Model file for the job. Use its own axes, mm. Face numbers are marked on the shaded views. A direction names the side the tool comes from. Coordinates: 2 decimals unless noted, no trailing zeros. Order: outer loops, then holes, each group sorted by start corner. A loop starts at its lowest first (then second) coordinate and runs counter-clockwise, first axis right, second up. Notation, with made-up numbers: M -34.5,31 L 3.5,31 A24 ccw 3.5,54 Z; hole C 33.25,48.25 d4. An arc over 180 degrees is marked long. Return JSON: item names as keys, results as strings.
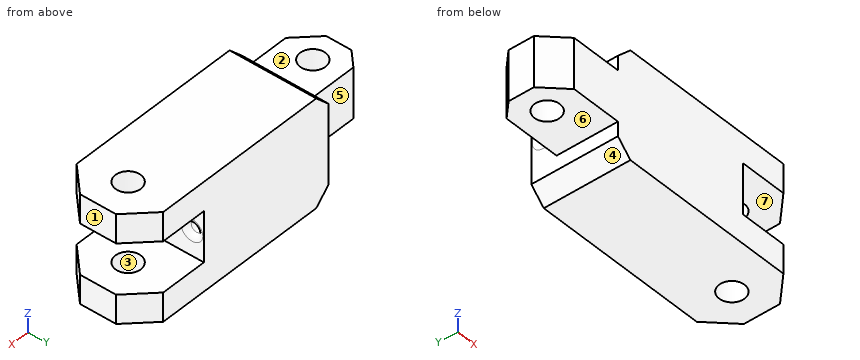
```python
from build123d import *

# Parameters (mm, degrees)
SKETCH_2_W            = 15
SKETCH_2_H            = 12
EXTRUDE_1_DEPTH       = 40
SKETCH_3_W            = 13.345049732
SKETCH_3_H            = 6.461251269
CUT_EXTRUDE_1_DEPTH   = 43.429353047
SKETCH_4_R            = 1.75
CUT_EXTRUDE_2_DEPTH   = 42.91658383
SKETCH_5_W            = 15.367688112
SKETCH_5_H            = 7
CUT_EXTRUDE_2_2_DEPTH = 43.429353047
CHAMFER_4_SIZE        = 3.5
SKETCH_7_R            = 0.75
CUT_EXTRUDE_3_DEPTH   = 32.5
CHAMFER_5_SIZE        = 3
SKETCH_8_W            = 20.918678204
SKETCH_8_H            = 3.864211738
CUT_EXTRUDE_4_DEPTH   = 10
CHAMFER_6_SIZE        = 2
SKETCH_9_R            = 1.75
CUT_EXTRUDE_5_DEPTH   = 44.13930922
FILLET_6_R            = 0.75
CHAMFER_7_SIZE        = 2


with BuildPart() as part:
    # Эскиз2 → Вытянуть1 (new body)
    with BuildSketch(Plane(origin=(0, 0, 0), x_dir=(0, 0, -1), z_dir=(1, 0, 0))):
        Rectangle(SKETCH_2_W, SKETCH_2_H)
    extrude(amount=EXTRUDE_1_DEPTH)

    # Эскиз3 → Вырез-Вытянуть1 (cut, through all)
    with BuildSketch(Plane(origin=(0, 6, 0), x_dir=(1, 0, 0), z_dir=(0, 1, 0))):
        with Locations((3.327475134, -6.730625634)):
            Rectangle(SKETCH_3_W, SKETCH_3_H)
        with Locations((3.327475134, 6.730625634)):
            Rectangle(SKETCH_3_W, SKETCH_3_H)
    extrude(amount=-CUT_EXTRUDE_1_DEPTH, mode=Mode.SUBTRACT)

    # Эскиз4 → Cut-Extrude 2 (cut, through all)
    with BuildSketch(Plane.XY.offset(3.5)):
        with Locations((3.849904433, -1.520907782)):
            Circle(SKETCH_4_R)
    extrude(amount=-CUT_EXTRUDE_2_DEPTH, mode=Mode.SUBTRACT)

    # Эскиз5 → Cut-Extrude 2 2 (cut, through all)
    with BuildSketch(Plane(origin=(0, 6, 0), x_dir=(1, 0, 0), z_dir=(0, 1, 0))):
        with Locations((37.683844056, 0)):
            Rectangle(SKETCH_5_W, SKETCH_5_H)
    extrude(amount=-CUT_EXTRUDE_2_2_DEPTH, mode=Mode.SUBTRACT)

    # Фаска4
    chamfer_4_edges = [part.edges().sort_by_distance(p)[0] for p in [
        (40, -6, 5.5),
        (40, 6, 5.5),
        (40, -6, -5.5),
        (40, 6, -5.5),
    ]]
    chamfer(chamfer_4_edges, length=CHAMFER_4_SIZE)

    # Эскиз7 → Вытянуть3 (cut, through all)
    with BuildSketch(Plane(origin=(30, 0, 0), x_dir=(0, 0, -1), z_dir=(1, 0, 0))):
        with Locations((0, 4.357693323)):
            Circle(SKETCH_7_R)
    extrude(amount=-CUT_EXTRUDE_3_DEPTH, mode=Mode.SUBTRACT)

    # Фаска5
    chamfer_5_edges = [part.edges().sort_by_distance(p)[0] for p in [
        (0, -6, 0),
    ]]
    chamfer(chamfer_5_edges, length=CHAMFER_5_SIZE)

    # Эскиз8 → Вытянуть4 (cut)
    with BuildSketch(Plane.ZY):
        with Locations((-0.939401822, 4.432105869)):
            Rectangle(SKETCH_8_W, SKETCH_8_H)
    extrude(amount=-CUT_EXTRUDE_4_DEPTH, mode=Mode.SUBTRACT)

    # Фаска6
    chamfer_6_edges = [part.edges().sort_by_distance(p)[0] for p in [
        (0, 2.5, 0),
    ]]
    chamfer(chamfer_6_edges, length=CHAMFER_6_SIZE)

    # Эскиз9 → Вытянуть5 (cut, through all)
    with BuildSketch(Plane.XY.offset(7.5)):
        with Locations((35.185724632, 0)):
            Circle(SKETCH_9_R)
    extrude(amount=-CUT_EXTRUDE_5_DEPTH, mode=Mode.SUBTRACT)

    # Скругление6
    fillet_6_edges = [part.edges().sort_by_distance(p)[0] for p in [
        (30, 4.357693323, 0.75),
        (10, 4.357693323, 0.75),
    ]]
    fillet(fillet_6_edges, radius=FILLET_6_R)

    # Фаска7
    chamfer_7_edges = [part.edges().sort_by_distance(p)[0] for p in [
        (10, 0, -7.5),
        (10, 0, 7.5),
    ]]
    chamfer(chamfer_7_edges, length=CHAMFER_7_SIZE)


solid = part.part
```
Item 1: Saw through at D-D (z = 6.75). Write the cut outline in (x, y), and give its area (3 significant figures).
Check result:
{"outline": "M 11.25,-6 L 36.5,-6 L 40,-2.5 L 40,2.5 L 36.5,6 L 11.25,6 Z; hole C 35.19,0 d3.5", "area": "323 mm2"}
Item 2: 3-axis set-ups, long thin cutter, end or side, ignore diameter. For the marked faces 5, 6 and 7: which of +Z, -Z, +X, -X, +Y, -Y reach the whole face in a straight line?
Check result:
{"face 5": "+Z, -Z, -X, +Y", "face 6": "-Z, -X, +Y, -Y", "face 7": "+X, +Y, -Y"}
Item 3: Saw through at B-B (z = -5). Write the cut outline in (x, y).
Check result:
{"outline": "M 10,-6 L 36.5,-6 L 40,-2.5 L 40,2.5 L 36.5,6 L 10,6 Z; hole C 35.19,0 d3.5"}
Item 4: Wall check: line 1 (Z direction, x = 31, y = -1.75); line 2 (Y direction, x = 19.5, z = 0); line 3 (X direction, y = 1.25, z = -0.5). Give the ranges that are in metal, low to high.
Check result:
{"line 1": "z = -7.5 to -3.5, 3.5 to 7.5", "line 2": "y = -6 to 3.61, 5.11 to 6", "line 3": "x = 0.75 to 30"}
Item 5: Saw through at C-C (z = 0). Write the cut outline in (x, y).
Check result:
{"outline": "M 0,-3 L 3,-6 L 30,-6 L 30,2.86 A0.75 ccw 29.25,3.61 L 10.75,3.61 A0.75 ccw 10,2.86 L 10,2.5 L 2,2.5 L 0,0.5 Z; M 10,5.86 A0.75 ccw 10.75,5.11 L 29.25,5.11 A0.75 ccw 30,5.86 L 30,6 L 10,6 Z; hole C 3.85,-1.52 d3.5"}
Item 6: Drop flat-ended pins along their axis: pin 1 Ø4 at (x, y) = (3.85, -1.52) entering from -Z; pin 2 Ø2 at (x, z) = (6.5, 1.5) entering from +Y; pin 3 Ø2 at (y, z) = (2.5, -1) entering from +X. Give the stop position or say it passes through.
Check result:
{"pin 1": "stops at z = -3.5", "pin 2": "stops at y = 2.5", "pin 3": "stops at x = 30"}
Item 7: Pull direction X, two halves, no side cores. Call the marked faces 1, 2, 3 and 4: +X half, -X half, draft (parallel to the pull), parting line (faces both ways), or undercut.
Check result:
{"face 1": "+X half", "face 2": "draft", "face 3": "undercut", "face 4": "-X half"}
Item 8: Saw through at A-A (x = 37.5). Write the cut outline in (y, z), and give its area (3 significant figures).
Check result:
{"outline": "M -5,-7.5 L 5,-7.5 L 5,-3.5 L -5,-3.5 Z; M -5,3.5 L 5,3.5 L 5,7.5 L -5,7.5 Z", "area": "80.0 mm2"}
